The model under review builds one solid part; all positions refer to its coordinate system, in mm. A direction names the side the tool comes from. Coordinates: 2 decimals unless noted, no trailing zeros. Write each loop counter-clockwise with the first axis right and the second up, starting at its lowest first coordinate (ties: lowest second). Pieces come first, ordered by that corner, then holes. Notation, with made-up numbers: (80.5, 70.25) -> (101.5, 70.25) arc R14 cw to (101.5, 84.25) -> close; hole circle Ø6 at (82, -24). An arc over 180 degrees is marked (long way). Write each question's results on one line, items separated by ' | '.
```python
from build123d import *

# Parameters (mm, degrees)
F0_W     = 220
F0_H     = 40
F1_DEPTH = 5
F2_W     = 120
F2_H     = 5
F3_DEPTH = 40
F4_W     = 40
F4_H     = 110
F5_DEPTH = 5
F6_W     = 5
F6_H     = 55
F7_DEPTH = 40
F8_R     = 4
F9_DEPTH = 25


with BuildPart() as f1:
    # F0 (on Top) → F1 (new body)
    with BuildSketch(Plane.XY):
        Rectangle(F0_W, F0_H)
    extrude(amount=F1_DEPTH)

    # F2 (on face) → F3 (join)
    with BuildSketch(Plane(origin=(0, 0, 0), x_dir=(1, 0, 0), z_dir=(0, 0, -1))):
        with Locations((-10, 17.5)):
            Rectangle(F2_W, F2_H)
    extrude(amount=F3_DEPTH)

    # F4 (on face) → F5 (join)
    with BuildSketch(Plane(origin=(0, 0, 0), x_dir=(1, 0, 0), z_dir=(0, 0, -1))):
        with Locations((-90, 75)):
            Rectangle(F4_W, F4_H)
    extrude(amount=-F5_DEPTH)

    # F6 (on face) → F7 (join)
    with BuildSketch(Plane(origin=(0, 0, 0), x_dir=(1, 0, 0), z_dir=(0, 0, -1))):
        with Locations((-72.5, 42.5)):
            Rectangle(F6_W, F6_H)
        Polygon((-75, 15), (-70, 15), (-70, 20), (-70, 70), (-75, 70), align=None)
    extrude(amount=F7_DEPTH)

    # F8 (on face) → F9 (cut)
    with BuildSketch(Plane.XY.offset(5)):
        with Locations((-95, -110)):
            Circle(F8_R)
        with Locations((85, 0)):
            Circle(F8_R)
    extrude(amount=-F9_DEPTH, mode=Mode.SUBTRACT)


solid = f1.part
```
Q1. Draft analysis for pull direction X (two halves, no side actions). For faces 1 (the flat face through (-1, -20, -18)), 2 (the cylindrical face through (-95.521, -106.034, 2.535)), 3 (the flat face through (110, 0, 2)), state which applies: pulls with the +X half, pulls with the -X half, needs draft (parallel to the pull), parting line crosses it, or undercut.
Solution:
face 1: needs draft | face 2: undercut | face 3: pulls with the +X half
Q2. Machinability: for faces 4 (the flat face through (-13, -15, -20)), 5 (the flat face through (-73, -70, -20)), 6 (the flat face through (-70, -50, -17)), 7 (the flat face through (-75, -42, -20)), which of the approach directions +Z, -Z, +X, -X, +Y, -Y give a long, thin tool a straight path to every point of the face, cutting with its end or side? Answer none if there is none.
Solution:
face 4: -Z, +X, -X, +Y | face 5: -Z, +X, -X, -Y | face 6: +Z, -Z, +X, -Y | face 7: -Z, -X, +Y, -Y
Q3. Clearance check with flat-ended pins moving along their axes: P1, Ø12, axis at x = 21, z = -5, coming from the -Y side; P2, Ø10, axis at y = -50.5, z = -25.5, coming from the +X side; P3, Ø1.5, axis at x = -23, z = -16.5, coming from the +Y side; P4, Ø5, axis at x = -95, y = -110, coming from the +Z side. State where each tip first meets the part, or that it passes through.
Solution:
P1: y = -20 | P2: x = -70 | P3: y = -15 | P4: through
Q4. For line 1 (Y direction, x = -95, z = 1.35); line 2 (Y direction, x = 85, z = 1); line 3 (Z direction, x = 14, y = -8.5), list the stretches that pass through material, from the lowest coordinate up. Write a range as from..to.
Solution:
line 1: -130..-114, -106..20 | line 2: -20..-4, 4..20 | line 3: 0..5
Q5. Add section C-C (z = -11.5). Write out the cut boundary in (x, y).
Solution:
outline: (-75, -70) -> (-70, -70) -> (-70, -20) -> (50, -20) -> (50, -15) -> (-75, -15) -> close
Q6. Add section B-B (y = -110). Write out the cut boundary in (x, z), plus the area to 3 significant figures.
Solution:
outline: (-110, 0) -> (-99, 0) -> (-99, 5) -> (-110, 5) -> close; (-91, 0) -> (-70, 0) -> (-70, 5) -> (-91, 5) -> close | area: 160 mm²
Q7. Add section A-A (x = -95). Write out the cut boundary in (y, z), plus the area to 3 significant figures.
Solution:
outline: (-130, 0) -> (-114, 0) -> (-114, 5) -> (-130, 5) -> close; (-106, 0) -> (20, 0) -> (20, 5) -> (-106, 5) -> close | area: 710 mm²
Q8. Add section D-D (x = -60). Write out the cut boundary in (y, z).
Solution:
outline: (-20, -40) -> (-15, -40) -> (-15, 0) -> (20, 0) -> (20, 5) -> (-20, 5) -> close
